Check sheet for the modelled part. Datum: model origin and axes. Units: mm. Face numbers are marked on the shaded views. A direction names the side the tool comes from. Coordinates: 2 decimals unless noted, no trailing zeros. Order: outer loops, then holes, each group sorted by start corner. A loop starts at its lowest first (then second) coordinate and runs counter-clockwise, first axis right, second up.
1. Cross-section at B-B (x = 2.45). Enter the section's corners in (y, z) (3 decimals), then the cut area to 3 significant figures.
2. Cross-section at C-C (y = 16.5). Enter the section's corners in (x, z), then the cut area to 3 significant figures.
3. Thickness scan on line 1 (Y direction, x = -2.15, z = 1.3) (3 decimals); line 2 (X direction, y = -17, z = 0.9). Record the ranges inside material, lowest first.
4. Gauge pin test, flat ends, axial feed: pin 1 Ø1.5 at (y, z) = (16.5, 1) entering from -X; pin 2 Ø0.5 at (x, z) = (2.5, 2) entering from -Y (3 decimals); pin 3 Ø0.5 at (x, z) = (2.5, 1) entering from +Y (3 decimals). Record the tip position at first contact, or that the pin passes through.
5. Set-up check for the marked faces 1, 2 and 3: record each of +Z, -Z, +X, -X, +Y, -Y from which the full face is reachable in a straight line by a thin tool's end or side.
6. Cross-section at A-A (z = 2). Enter the section's corners in (x, y) (3 decimals).
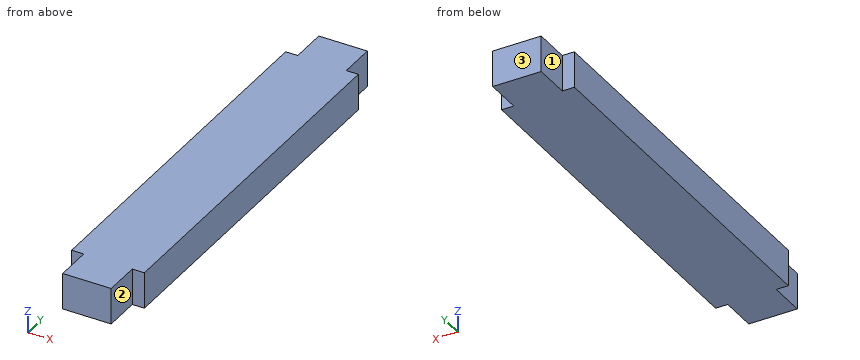
Autodesk Inventor part; units mm, degrees
ref_plane "YZ Plane" through (0, 0, 0) normal (1, 0, 0) x (0, 1, 0)
ref_plane "XZ Plane" through (0, 0, 0) normal (0, 1, 0) x (-1, 0, 0)
ref_plane "XY Plane" through (0, 0, 0) normal (0, 0, 1) x (1, 0, 0)
sketch "Sketch1" plane through (0, 0, 0) normal (0, 0, 1) x (1, 0, 0)
  line L0 (-3, 15.255) -> (3, 15.255)
  line L1 (3, 15.255) -> (3, -15.255)
  line L2 (3, -15.255) -> (-3, -15.255)
  line L3 (-3, -15.255) -> (-3, 15.255)
  line L4 (-2, -15.255) -> (2, -15.255)
  line L5 (2, -15.255) -> (2, -18.255)
  line L6 (2, -18.255) -> (-2, -18.255)
  line L7 (-2, -18.255) -> (-2, -15.255)
  line L8 (-2, 15.255) -> (2, 15.255)
  line L9 (2, 15.255) -> (2, 18.255)
  line L10 (2, 18.255) -> (-2, 18.255)
  line L11 (-2, 18.255) -> (-2, 15.255)
  line L12 (3, -12) -> (0, -12)
  line L13 (0, -12) -> (0, -8)
  line L14 (0, -8) -> (3, -8)
  line L15 (3, -8) -> (3, -12)
  line L16 (3, 8) -> (0, 8)
  line L17 (0, 8) -> (0, 12)
  line L18 (0, 12) -> (3, 12)
  line L19 (3, 12) -> (3, 8)
  point P0 (0, 0)
  point P1 (0, 0)
  point P2 (0, 18.255)
  point P3 (0, 15.255)
  point P4 (0, 15.255)
  point P5 (0, -18.255)
  point P6 (3, 0)
  point P7 (2.1852, -20.4852)
  point P8 (2.1852, 20.1148)
  point P9 (3, -10)
  point P10 (3, 10)
  point P11 (3.1852, -8.1852)
  point P12 (3.1852, 11.8148)
  dimension "d0" = 36.51
  dimension "d1" = 3
  dimension "d2" = 4
  dimension "d3" = 6
  dimension "d4" = 4
  dimension "d5" = 10
  dimension "d6" = 10
  dimension "d7" = 3
extrude "Extrusion1" add sketch "Sketch1" along normal blind 3
properties material "MDF Medium Density Fiberboard"
Data:
1. outline: (-15.255, 0) - (15.255, 0) - (15.255, 3) - (-15.255, 3) - close
1. area: 91.5 mm2
2. outline: (-2, 0) - (2, 0) - (2, 3) - (-2, 3) - close
2. area: 12.0 mm2
3. line 1: y = -15.255 to 15.255
3. line 2: x = -2 to 2
4. pin 1: stops at x = -2
4. pin 2: stops at y = -15.255
4. pin 3: stops at y = 15.255
5. face 1: +Z, -Z, -X, +Y
5. face 2: +Z, -Z, +X, -Y
5. face 3: +Z, -Z, +X, -X, +Y
6. outline: (-3, -15.255) - (-2, -15.255) - (-2, -18.255) - (2, -18.255) - (2, -15.255) - (3, -15.255) - (3, 15.255) - (2, 15.255) - (2, 18.255) - (-2, 18.255) - (-2, 15.255) - (-3, 15.255) - close
